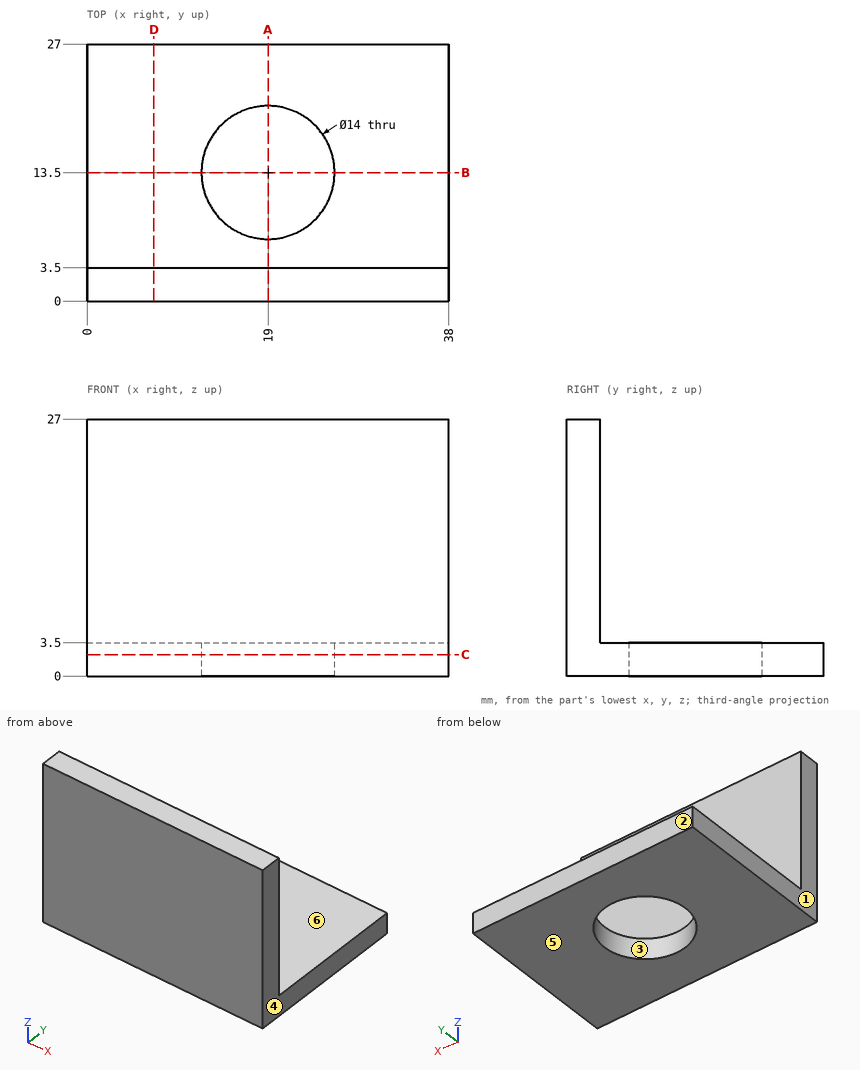
Print and shaded views of the part. All mm, measured from the part's lowest x, y and z. A direction names the side the tool comes from. Coordinates: 2 decimals unless noted, no trailing zeros. Order: outer loops, then holes, each group sorted by start corner. A loop starts at its lowest first (then second) coordinate and runs counter-clockwise, first axis right, second up. Notation, with made-up numbers: (-8, 2.5) -> (20, 2.5) arc R23 cw to (20, 24.5) -> close; hole circle Ø5 at (81, 16.5). An arc over 180 degrees is marked (long way). Use one line per item in the form item = value. Start each with the question number.
1) Drop a flat-ended pin along its axis: pin 1 (12 mm diameter, centred on x = 24, z = 19, fed in from +Y). Give the stop position or say it passes through.
2) Band-saw the part on B-B on y = 13.5. Give the cut face in (x, z), then the cut area to 3 significant figures.
3) Pull direction X, two halves, no side cores. Call the marked faces 1, 2, 3 and 4: +X half, -X half, draft (parallel to the pull), parting line (faces both ways), or undercut.
4) Drill centre lines: L1, parallel to Y at x = 19, z = 2; L2, parallel to Y at x = 29.5, z = 6.25. Where is each one in solid material? Low to high. Write a range as [from, to].
5) Tool access for the marked faces 5 and 6: list every direction of +Z, -Z, +X, -X, +Y, -Y with a clear straight run to the whole face (end or side of a thin tool).
6) Band-saw the part on A-A on x = 19. Give the cut face in (y, z).
7) Band-saw the part on D-D on x = 7. Give the cut face in (y, z).
8) Band-saw the part on C-C on z = 2.25. Give the cut face in (x, y), then the cut area to 3 significant figures.
Entries:
q1.pin_1 = 3.5
q2.outline = (0, 0) -> (12, 0) -> (12, 3.5) -> (0, 3.5) -> close; (26, 0) -> (38, 0) -> (38, 3.5) -> (26, 3.5) -> close
q2.area = 84.0 mm2
q3.face_1 = -X half
q3.face_2 = draft
q3.face_3 = undercut
q3.face_4 = +X half
q4.L1 = [0, 6.5], [20.5, 27]
q4.L2 = [0, 3.5]
q5.face_5 = -Z, +X, -X, +Y, -Y
q5.face_6 = +Z, +X, -X, +Y
q6.outline = (0, 0) -> (6.5, 0) -> (6.5, 3.5) -> (3.5, 3.5) -> (3.5, 27) -> (0, 27) -> close; (20.5, 0) -> (27, 0) -> (27, 3.5) -> (20.5, 3.5) -> close
q7.outline = (0, 0) -> (27, 0) -> (27, 3.5) -> (3.5, 3.5) -> (3.5, 27) -> (0, 27) -> close
q8.outline = (0, 0) -> (38, 0) -> (38, 27) -> (0, 27) -> close; hole circle Ø14 at (19, 13.5)
q8.area = 872 mm2
